```python
from build123d import *

# Parameters (mm, degrees)
SKETCH1_W            = 93.4
SKETCH1_H            = 17.2
SKETCH1_R            = 2.5
SKETCH1_R_2          = 6
SKETCH1_W_2          = 12
SKETCH1_H_2          = 12
SKETCH1_H_3          = 70
SKETCH1_R_3          = 1.45
SKETCH1_W_3          = 6.5
SKETCH1_H_4          = 43
SKETCH1_W_4          = 78.25
SKETCH1_H_5          = 51
SKETCH1_R_4          = 3.5
BOSS_EXTRUDE2_DEPTH  = 1.57
BOSS_EXTRUDE3_START  = 4.6
SKETCH1_3_W          = 93.4
SKETCH1_3_H          = 70
SKETCH1_3_R          = 1.45
BOSS_EXTRUDE3_DEPTH  = 4.6
SKETCH1_4_W          = 78.25
SKETCH1_4_H          = 51
BOSS_EXTRUDE4_DEPTH  = 14.4
SKETCH1_5_W          = 6.5
SKETCH1_5_H          = 43
BOSS_EXTRUDE5_DEPTH  = 9.7
SKETCH1_6_W          = 12
SKETCH1_6_H          = 12
BOSS_EXTRUDE6_DEPTH  = 7
SKETCH1_7_R          = 3.5
BOSS_EXTRUDE7_DEPTH  = 27
SKETCH1_8_R          = 6
BOSS_EXTRUDE8_DEPTH  = 9.3
SKETCH1_9_R          = 2.5
BOSS_EXTRUDE9_DEPTH  = 5.1
SKETCH3_W            = 26.26
SKETCH3_H            = 26.47
BOSS_EXTRUDE10_DEPTH = 4
SKETCH4_W            = 20.28
SKETCH4_H            = 9
BOSS_EXTRUDE11_DEPTH = 20
CUT_EXTRUDE1_DEPTH   = 1
SKETCH6_W            = 26.47
SKETCH6_H            = 4
CUT_EXTRUDE2_DEPTH   = 1
SKETCH7_W            = 7
SKETCH7_H            = 7
BOSS_EXTRUDE12_DEPTH = 10


with BuildPart() as part:
    # Sketch1 → Boss-Extrude2 (new body)
    # profile 1 of 8: a face of its own
    with BuildSketch(Plane(origin=(0, 0, 0), x_dir=(1, 0, 0), z_dir=(0, 1, 0))):
        with Locations((0, -35)):
            Rectangle(SKETCH1_W, SKETCH1_H)
        with Locations((3.2, -34.6)):
            Circle(SKETCH1_R, mode=Mode.SUBTRACT)
        with Locations((18.2, -34.6)):
            Circle(SKETCH1_R_2, mode=Mode.SUBTRACT)
        with Locations((36.7, -34.6)):
            Rectangle(SKETCH1_W_2, SKETCH1_H_2, mode=Mode.SUBTRACT)
    # profile 2 of 8: a face of its own
    with BuildSketch(Plane(origin=(0, 0, 0), x_dir=(1, 0, 0), z_dir=(0, 1, 0))):
        with Locations((0, 8.6)):
            Rectangle(SKETCH1_W, SKETCH1_H_3)
        with Locations(Location((-44.2, -23.9, 0), (0, 0, 270))):
            Circle(SKETCH1_R_3, mode=Mode.SUBTRACT)
        with Locations(Location((44.2, -23.9, 0), (0, 0, 270))):
            Circle(SKETCH1_R_3, mode=Mode.SUBTRACT)
        Polygon((-39.125, 32.527837259), (-39.125, 36.527837259), (39.125, 36.527837259), (39.125, -14.472162741), (-39.125, -14.472162741), (-39.125, -10.472162741), (-45.625, -10.472162741), (-45.625, 32.527837259), align=None, mode=Mode.SUBTRACT)
        with Locations(Location((-44.2, 41.1, 0), (0, 0, 270))):
            Circle(SKETCH1_R_3, mode=Mode.SUBTRACT)
        with Locations(Location((44.2, 41.1, 0), (0, 0, 270))):
            Circle(SKETCH1_R_3, mode=Mode.SUBTRACT)
    # profile 3 of 8: a face of its own
    with BuildSketch(Plane(origin=(0, 0, 0), x_dir=(1, 0, 0), z_dir=(0, 1, 0))):
        with Locations((-42.375, 11.027837259)):
            Rectangle(SKETCH1_W_3, SKETCH1_H_4)
    # profile 4 of 8: a face of its own
    with BuildSketch(Plane(origin=(0, 0, 0), x_dir=(1, 0, 0), z_dir=(0, 1, 0))):
        with Locations((0, 11.027837259)):
            Rectangle(SKETCH1_W_4, SKETCH1_H_5)
    # profile 5 of 8: a face of its own
    with BuildSketch(Plane(origin=(0, 0, 0), x_dir=(1, 0, 0), z_dir=(0, 1, 0))):
        with Locations((3.2, -34.6)):
            Circle(SKETCH1_R)
    # profile 6 of 8: a face of its own
    with BuildSketch(Plane(origin=(0, 0, 0), x_dir=(1, 0, 0), z_dir=(0, 1, 0))):
        with Locations((18.2, -34.6)):
            Circle(SKETCH1_R_2)
    # profile 7 of 8: a face of its own
    with BuildSketch(Plane(origin=(0, 0, 0), x_dir=(1, 0, 0), z_dir=(0, 1, 0))):
        with Locations((36.7, -34.6)):
            Rectangle(SKETCH1_W_2, SKETCH1_H_2)
        with Locations((36.7, -34.6)):
            Circle(SKETCH1_R_4, mode=Mode.SUBTRACT)
    # profile 8 of 8: a face of its own
    with BuildSketch(Plane(origin=(0, 0, 0), x_dir=(1, 0, 0), z_dir=(0, 1, 0))):
        with Locations((36.7, -34.6)):
            Circle(SKETCH1_R_4)
    extrude(amount=-BOSS_EXTRUDE2_DEPTH)

    # Sketch1_3 → Boss-Extrude3 (add)
    with BuildSketch(Plane(origin=(0, 0, 0), x_dir=(1, 0, 0), z_dir=(0, 1, 0)).offset(BOSS_EXTRUDE3_START)):
        with Locations((0, 8.6)):
            Rectangle(SKETCH1_3_W, SKETCH1_3_H)
        with Locations((-44.2, -23.9)):
            Circle(SKETCH1_3_R, mode=Mode.SUBTRACT)
        with Locations((44.2, -23.9)):
            Circle(SKETCH1_3_R, mode=Mode.SUBTRACT)
        with Locations((-44.2, 41.1)):
            Circle(SKETCH1_3_R, mode=Mode.SUBTRACT)
        with Locations((44.2, 41.1)):
            Circle(SKETCH1_3_R, mode=Mode.SUBTRACT)
    extrude(amount=-BOSS_EXTRUDE3_DEPTH)

    # Sketch1_4 → Boss-Extrude4 (add)
    with BuildSketch(Plane(origin=(0, 0, 0), x_dir=(1, 0, 0), z_dir=(0, 1, 0))):
        with Locations((0, 11.027837259)):
            Rectangle(SKETCH1_4_W, SKETCH1_4_H)
    extrude(amount=BOSS_EXTRUDE4_DEPTH)

    # Sketch1_5 → Boss-Extrude5 (add)
    with BuildSketch(Plane(origin=(0, 0, 0), x_dir=(1, 0, 0), z_dir=(0, 1, 0))):
        with Locations((-42.375, 11.027837259)):
            Rectangle(SKETCH1_5_W, SKETCH1_5_H)
    extrude(amount=BOSS_EXTRUDE5_DEPTH)

    # Sketch1_6 → Boss-Extrude6 (add)
    with BuildSketch(Plane(origin=(0, 0, 0), x_dir=(1, 0, 0), z_dir=(0, 1, 0))):
        with Locations((36.7, -34.6)):
            Rectangle(SKETCH1_6_W, SKETCH1_6_H)
    extrude(amount=BOSS_EXTRUDE6_DEPTH)

    # Sketch1_7 → Boss-Extrude7 (add)
    with BuildSketch(Plane(origin=(0, 0, 0), x_dir=(1, 0, 0), z_dir=(0, 1, 0))):
        with Locations(Location((36.7, -34.6, 0), (0, 0, 270))):
            Circle(SKETCH1_7_R)
    extrude(amount=BOSS_EXTRUDE7_DEPTH)

    # Sketch1_8 → Boss-Extrude8 (add)
    with BuildSketch(Plane(origin=(0, 0, 0), x_dir=(1, 0, 0), z_dir=(0, 1, 0))):
        with Locations(Location((18.2, -34.6, 0), (0, 0, 270))):
            Circle(SKETCH1_8_R)
    extrude(amount=BOSS_EXTRUDE8_DEPTH)

    # Sketch1_9 → Boss-Extrude9 (add)
    with BuildSketch(Plane(origin=(0, 0, 0), x_dir=(1, 0, 0), z_dir=(0, 1, 0))):
        with Locations(Location((3.2, -34.6, 0), (0, 0, 270))):
            Circle(SKETCH1_9_R)
    extrude(amount=BOSS_EXTRUDE9_DEPTH)

    # Sketch3 → Boss-Extrude10 (add)
    with BuildSketch(Plane.XZ.offset(1.57)):
        with Locations((-33.57, -8.405)):
            Rectangle(SKETCH3_W, SKETCH3_H)
    extrude(amount=BOSS_EXTRUDE10_DEPTH)

    # Sketch4 → Boss-Extrude11 (add)
    with BuildSketch(Plane.XZ.offset(1.57)):
        with Locations((-15.18, -32.7)):
            Rectangle(SKETCH4_W, SKETCH4_H)
        with Locations((15.44, -32.7)):
            Rectangle(SKETCH4_W, SKETCH4_H)
    extrude(amount=BOSS_EXTRUDE11_DEPTH)

    # Sketch5 → Cut-Extrude1 (cut)
    with BuildSketch(Plane(origin=(0, 14.4, 0), x_dir=(1, 0, 0), z_dir=(0, 1, 0))):
        with BuildLine():
            Line((33.625, 30.677837259), (-33.625, 30.677837259))
            ThreePointArc((-33.625, 30.677837259), (-35.039213562, 30.092050821), (-35.625, 28.677837259))
            Line((-35.625, 28.677837259), (-35.625, -6.622162741))
            ThreePointArc((-35.625, -6.622162741), (-35.039213562, -8.036376303), (-33.625, -8.622162741))
            Line((-33.625, -8.622162741), (33.625, -8.622162741))
            ThreePointArc((33.625, -8.622162741), (35.039213562, -8.036376303), (35.625, -6.622162741))
            Line((35.625, -6.622162741), (35.625, 28.677837259))
            ThreePointArc((35.625, 28.677837259), (35.039213562, 30.092050821), (33.625, 30.677837259))
        make_face()
    extrude(amount=-CUT_EXTRUDE1_DEPTH, mode=Mode.SUBTRACT)

    # Sketch6 → Cut-Extrude2 (cut)
    with BuildSketch(Plane.ZY.offset(46.7)):
        with Locations((-8.405, -3.57)):
            Rectangle(SKETCH6_W, SKETCH6_H)
    extrude(amount=-CUT_EXTRUDE2_DEPTH, mode=Mode.SUBTRACT)

    # Sketch7 → Boss-Extrude12 (add)
    with BuildSketch(Plane(origin=(0, 0, 0), x_dir=(1, 0, 0), z_dir=(0, 1, 0))):
        with Locations((-38.2, -32.1)):
            Rectangle(SKETCH7_W, SKETCH7_H)
    extrude(amount=BOSS_EXTRUDE12_DEPTH)


solid = part.part
```
Geometry: final body of the model. Coordinates: model frame, mm. A direction names the side the tool comes from. Coordinates: 2 decimals unless noted, no trailing zeros. Loops run counter-clockwise (first coordinate to the right, second up) from the corner with the lowest first, then second, coordinate; pieces in that order, holes last. Notation, with made-up numbers: (3, 83.5) -> (23, 83.5) arc R24 ccw to (23, 97.5) -> close; hole circle Ø1 at (40, -7). An arc over 180 degrees is marked (long way). Use a Markdown table: item, result. Add a question column.
(1) Line query: line 1 along X through (y, z) = (0.75, 23.9); line 2 along Z through (x, y) = (-44, 3); line 3 along Z through (x, y) = (-0.5, 13.5). Output: solid intervals per line, ascending.
(2) Mould query, pull axis X, two halves, no side actions, for faces 1 (the flat face through (-1, 2, 26.4)), 2 (the flat face through (-41.7, 5, 32)), 3 (the flat face through (-34.7, 5, 32)). Classes: pulls with the +X half, pulls with the -X half, needs draft (parallel to the pull), parting line crosses it, or undercut.
(3) Section query C-C, the plane x = 3.2. Return loops of the section in (y, z).
(4) Section query A-A, the plane z = -34. Return loops of the section in (x, y) (3 decimals), plus the area to 3 significant figures.
(5) Pin query (flat end, axial travel): pin 1 Ø1.5 at (x, y) = (-43.5, 7) entering from -Z; pin 2 Ø7.5 at (x, z) = (-34.5, -12.5) entering from -Y; pin 3 Ø6 at (x, z) = (32, -34.5) entering from +Y. Return the tip coordinate at first contact, or that it passes through.
(6) Section query B-B, the plane y = -17. Return loops of the section in (x, z), plus the area to 3 significant figures.
(7) Access query for faces 4 (the flat face through (30.7, 3, 35)), 5 (the flat face through (37, 3, 40.6)), 6 (the flat face through (39.125, 9, -11)), 7 (the flat face through (-42, 7, -32.528)). Directions: +Z, -Z, +X, -X, +Y, -Y. A direction counts if a zero-diameter tool reaches every point of the face in a straight line with its end or side. Return the directions, or none.
(8) Section query D-D, the plane z = -13.5. Return loops of the section in (x, y) (3 decimals), plus the area to 3 significant figures.
Answer:
| question | item | result |
|---|---|---|
| 1 | line 1 | x = -46.7 to -45.65, -42.75 to 42.75, 45.65 to 46.7 |
| 1 | line 2 | z = -43.6 to -42.54, -39.66 to 22.46, 25.34 to 26.4 |
| 1 | line 3 | z = -36.53 to -30.68, 8.62 to 14.47 |
| 2 | face 1 | needs draft |
| 2 | face 2 | pulls with the -X half |
| 2 | face 3 | undercut |
| 3 | outline | (-1.57, -43.6) -> (4.6, -43.6) -> (4.6, -36.53) -> (14.4, -36.53) -> (14.4, -30.68) -> (13.4, -30.68) -> (13.4, 8.62) -> (14.4, 8.62) -> (14.4, 14.47) -> (4.6, 14.47) -> (4.6, 26.4) -> (0, 26.4) -> (0, 32.1) -> (5.1, 32.1) -> (5.1, 37.1) -> (0, 37.1) -> (0, 43.6) -> (-1.57, 43.6) -> close |
| 4 | outline | (-46.7, -1.57) -> (-25.32, -1.57) -> (-25.32, -21.57) -> (-5.04, -21.57) -> (-5.04, -1.57) -> (5.3, -1.57) -> (5.3, -21.57) -> (25.58, -21.57) -> (25.58, -1.57) -> (46.7, -1.57) -> (46.7, 4.6) -> (39.125, 4.6) -> (39.125, 14.4) -> (-39.125, 14.4) -> (-39.125, 4.6) -> (-46.7, 4.6) -> close |
| 4 | area | 2,150 mm^2 |
| 5 | pin 1 | stops at z = -32.53 |
| 5 | pin 2 | stops at y = -5.57 |
| 5 | pin 3 | stops at y = 14.4 |
| 6 | outline | (-25.32, -37.2) -> (-5.04, -37.2) -> (-5.04, -28.2) -> (-25.32, -28.2) -> close; (5.3, -37.2) -> (25.58, -37.2) -> (25.58, -28.2) -> (5.3, -28.2) -> close |
| 6 | area | 365 mm^2 |
| 7 | face 4 | +Z, +Y |
| 7 | face 5 | +Z, +X, -X, +Y |
| 7 | face 6 | -Z, +X, +Y |
| 7 | face 7 | -Z, -X, +Y |
| 8 | outline | (-46.7, -1.57) -> (-45.7, -1.57) -> (-45.7, -5.57) -> (-20.44, -5.57) -> (-20.44, -1.57) -> (46.7, -1.57) -> (46.7, 4.6) -> (39.125, 4.6) -> (39.125, 14.4) -> (35.625, 14.4) -> (35.625, 13.4) -> (-35.625, 13.4) -> (-35.625, 14.4) -> (-39.125, 14.4) -> (-39.125, 9.7) -> (-45.625, 9.7) -> (-45.625, 4.6) -> (-46.7, 4.6) -> close |
| 8 | area | 1,410 mm^2 |
